Input: part model. Units: mm. Frame: model coordinates. A direction names the side the tool comes from. Coordinates: 2 decimals unless noted, no trailing zeros. Write each loop counter-clockwise with the first axis right and the second up, starting at its lowest first coordinate (ties: lowest second). Pieces come first, ordered by that corner, then holes. Notation, with made-up numbers: M 40,63 L 56,63 A25 cw 56,102 Z; hole C -23,-31 d4. An arc over 180 degrees is marked long. Write each question's results on one line, items separated by ' | '. Start each with the question number.
1. Section query D-D, the plane y = 14.75. Count the separate pieces of the cut face and the enclosed holes in it, and give its area (3 significant figures).
2. Set-up query: faces 4 (the flat face through (-26, 39.75, -2)), 5 (the flat face through (-46, -2, -99)), 6 (the flat face through (-4, 0, -4)). Return all of +Z, -Z, +X, -X, +Y, -Y with unobstructed straight access to the full face (end or side cutting, diameter ignored); none if empty.
3. Section query A-A, the plane x = -69.5. Output: boundary loops of the cut face in (y, z).
4. Section query C-C, the plane x = -50. Output: boundary loops of the cut face in (y, z), and give its area (3 significant figures).
5. First-contact query: pin 1 (8 mm diameter, centred on x = -46, z = -67, fed in from +Y); pin 2 (20 mm diameter, centred on x = -63.49, y = 14.75, fed in from +Z). Flat tips, straight axial feed; report the tip coordinate or a pass-through.
6. Pull-direction query (X, two-part tool) for faces 1 (the flat face through (-90, 29, -101)), 2 (the flat face through (-44, 29, -200)), 3 (the flat face through (-27, 48.75, -2)); classes: +X half, -X half, draft (parallel to the pull), parting line (faces both ways), or undercut.
7. Section query B-B, the plane z = -116.5. Output: boundary loops of the cut face in (x, y).
8. Ray query, probe 1 along X at (y, z) = (45, -196); probe 2 along Z at (x, y) = (-45.5, 1); probe 3 along X at (y, z) = (21.5, -57). Return the intervals inside material, ascending.
Autodesk Inventor part; units mm, degrees
ref_plane "YZ Plane" through (0, 0, 0) normal (1, 0, 0) x (0, 1, 0)
ref_plane "XZ Plane" through (0, 0, 0) normal (0, 1, 0) x (-1, 0, 0)
ref_plane "XY Plane" through (0, 0, 0) normal (0, 0, 1) x (1, 0, 0)
sketch "Sketch2" plane through (0, 0, 0) normal (0, 1, 0) x (-1, 0, 0)
  line L0 (0, 0) -> (0, -200)
  line L1 (0, -200) -> (90, -200)
  line L2 (90, -200) -> (90, 0)
  line L3 (90, 0) -> (0, 0)
  line L4 (0, 0) -> (0, -8)
  line L5 (2, -96) -> (8, -96)
  line L6 (8, -96) -> (8, -104)
  line L7 (8, -104) -> (2, -104)
  line L8 (2, -104) -> (2, -192)
  line L9 (2, -192) -> (8, -192)
  line L10 (8, -192) -> (8, -198)
  line L11 (8, -198) -> (45, -198)
  line L12 (8, -4) -> (45, -4)
  line L13 (8, -4) -> (8, -8)
  line L14 (88, -96) -> (82, -96)
  line L15 (82, -96) -> (82, -104)
  line L16 (82, -104) -> (88, -104)
  line L17 (88, -104) -> (88, -192)
  line L18 (88, -192) -> (82, -192)
  line L19 (82, -192) -> (82, -198)
  line L20 (82, -198) -> (45, -198)
  line L21 (82, -4) -> (45, -4)
  line L22 (82, -4) -> (82, -8)
  line L23 (90, -200) -> (90, -196)
  line L24 (0, -200) -> (0, -196)
  circle A0 centre (4, -196) radius 2.1
  circle A1 centre (86, -196) radius 2.1
  circle A2 centre (86, -100) radius 2.1
  circle A3 centre (86, -4) radius 2.1
  circle A4 centre (4, -4) radius 2.1
  circle A5 centre (4, -100) radius 2.1
  line L25 (6, -86) -> (6, -83)
  line L26 (6, -86) -> (2, -86)
  line L27 (2, -86) -> (2, -96)
  line L28 (6, -83) -> (2, -83)
  line L29 (2, -83) -> (2, -80)
  line L30 (2, -80) -> (6, -80)
  line L31 (6, -80) -> (6, -77)
  line L32 (6, -77) -> (2, -77)
  line L33 (84, -86) -> (84, -83)
  line L34 (84, -86) -> (88, -86)
  line L35 (84, -83) -> (88, -83)
  line L36 (88, -83) -> (88, -80)
  line L37 (88, -80) -> (84, -80)
  line L38 (84, -80) -> (84, -77)
  line L39 (84, -77) -> (88, -77)
  line L40 (88, -86) -> (88, -96)
  line L41 (84, -8) -> (84, -11)
  line L42 (84, -11) -> (88, -11)
  line L43 (88, -50) -> (84, -50)
  line L44 (84, -50) -> (84, -53)
  line L45 (84, -53) -> (88, -53)
  line L46 (82, -8) -> (84, -8)
  line L47 (88, -11) -> (88, -50)
  line L48 (88, -53) -> (88, -77)
  line L49 (6, -8) -> (6, -11)
  line L50 (6, -11) -> (2, -11)
  line L51 (2, -50) -> (6, -50)
  line L52 (6, -50) -> (6, -53)
  line L53 (6, -53) -> (2, -53)
  line L54 (8, -8) -> (6, -8)
  line L55 (2, -11) -> (2, -50)
  line L56 (2, -53) -> (2, -77)
  dimension "d1" = 200
  dimension "d2" = 90
  dimension "d3" = 200
  dimension "d4" = 8
  dimension "d5" = 8
  dimension "d8" = 6
  dimension "d9" = 8
  dimension "d10" = 6
  dimension "d11" = 88
  dimension "d12" = 6
  dimension "d13" = 6
  dimension "d41" = 4
  dimension "d43" = 4
  dimension "d45" = 4.2
  dimension "d46" = 4.2
  dimension "d47" = 4.2
  dimension "d48" = 4.2
  dimension "d49" = 4.2
  dimension "d50" = 4.2
  dimension "d87" = 3
  dimension "d88" = 4
  dimension "d89" = 4
  dimension "d90" = 3
  dimension "d92" = 4
  dimension "d93" = 3
  dimension "d94" = 4
  dimension "d96" = 3
  dimension "d98" = 3
extrude "Extrusion1" add sketch "Sketch2" along normal blind 59
sketch "Sketch11" plane through (-90, 0, 0) normal (0, 0, 1) x (1, 0, 0)
  circle A0 centre (26.5144, 14.75) radius 11
  line L0 (63.5431, 48.75) -> (72.5431, 48.75)
  line L1 (72.5431, 48.75) -> (72.5431, 39.75)
  line L2 (72.5431, 39.75) -> (54.5431, 39.75)
  line L3 (54.5431, 39.75) -> (54.5431, 48.75)
  line L4 (54.5431, 48.75) -> (63.5431, 48.75)
  dimension "d76" = 22
  dimension "d78" = 9
  dimension "d79" = 9
  dimension "d80" = 18
  dimension "d81" = 9
extrude "Extrusion7" cut sketch "Sketch11" against normal blind 5
sketch "Sketch12" plane through (0, 59, 0) normal (0, 1, 0) x (1, 0, 0)
  point P0 (0, 0)
sketch "Sketch13" plane through (-84, 0, -86) normal (0, 0, -1) x (-1, 0, 0)
  line L0 (0, 35) -> (4, 35)
  line L1 (0, 35) -> (0, 59)
  line L2 (0, 59) -> (4, 59)
  line L3 (0, 59) -> (4, 59)
  line L4 (4, 59) -> (4, 35)
  point P0 (-84, 0)
  point P1 (4, 0)
  point P2 (0, 0)
extrude "Extrusion8" cut sketch "Sketch13" against normal blind 78
sketch "Sketch14" plane through (-2, 0, -86) normal (0, 0, -1) x (-1, 0, 0)
  line L0 (4, 0) -> (4, 59)
  line L1 (4, 0) -> (4, 35)
  line L2 (4, 0) -> (39, 0) construction
  line L3 (4, 35) -> (0, 35)
  line L4 (0, 0) -> (0, 59)
  line L5 (0, 35) -> (0, 59)
  line L6 (0, 59) -> (4, 59)
  line L7 (4, 59) -> (4, 35)
  point P0 (-2, 0)
  dimension "d104" = 35
  dimension "d105" = 90
extrude "Extrusion9" cut sketch "Sketch14" against normal blind 78
sketch "Sketch15" plane through (0, 0, 0) normal (0, -1, 0) x (1, 0, 0)
  line L0 (-90, 0) -> (0, 0)
  line L1 (0, -200) -> (-90, -200)
  line L2 (0, 0) -> (0, -200)
  line L3 (0, -200) -> (-90, -200)
  line L4 (-90, -200) -> (-90, 0)
  line L5 (-90, 0) -> (0, 0)
extrude "Extrusion10" add sketch "Sketch15" along normal blind 2
properties part number "Housing Rev 3"
Answer:
1) separate pieces: 1 | enclosed holes: 6 | area: 1,460 mm^2
2) face 4: +Z | face 5: +Z, -Z, +X, -X, -Y | face 6: +Y
3) outline: M -2,-200 L 59,-200 L 59,-198 L 0,-198 L 0,-4 L 5.54,-4 L 5.54,0 L -2,0 Z; M 23.96,-4 L 59,-4 L 59,0 L 23.96,0 Z
4) outline: M -2,-200 L 59,-200 L 59,-198 L 0,-198 L 0,-4 L 59,-4 L 59,0 L -2,0 Z | area: 754 mm^2
5) pin 1: y = 0 | pin 2: z = -198
6) face 1: -X half | face 2: draft | face 3: undercut
7) outline: M -90,-2 L 0,-2 L 0,59 L -2,59 L -2,0 L -88,0 L -88,59 L -90,59 Z
8) probe 1: -90 to -88.1, -83.9 to -82, -8 to -6.1, -1.9 to 0 | probe 2: -200 to -198, -4 to 0 | probe 3: -90 to -88, -2 to 0
